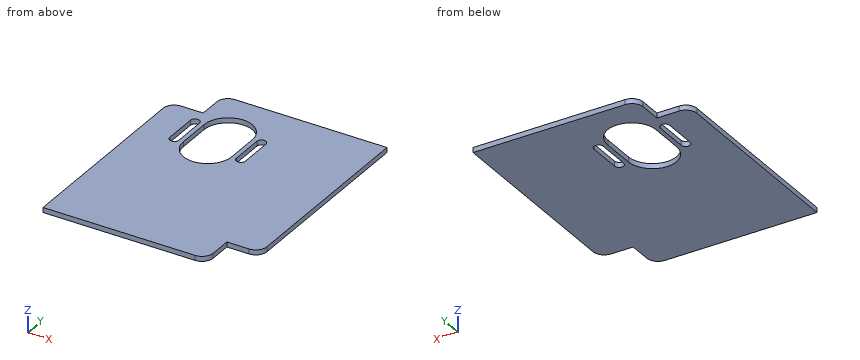
```python
from build123d import *

# Parameters (mm, degrees)
SKETCH1_W           = 118.275
SKETCH1_H           = 143.74
BOSS_EXTRUDE1_DEPTH = 3
CUT_EXTRUDE1_DEPTH  = 3
SKETCH3_W           = 20
SKETCH3_H           = 20
CUT_EXTRUDE2_DEPTH  = 10
FILLET1_R           = 6.7


with BuildPart() as part:
    # Sketch1 → Boss-Extrude1 (new body)
    with BuildSketch(Plane.XY):
        with Locations((59.1375, 71.87)):
            Rectangle(SKETCH1_W, SKETCH1_H)
    extrude(amount=BOSS_EXTRUDE1_DEPTH)

    # Sketch2 → Cut-Extrude1 (cut)
    with BuildSketch(Plane.XY.offset(3)):
        with BuildLine():
            Line((55.5, 114.05), (55.5, 94.05))
            ThreePointArc((55.5, 94.05), (41, 79.55), (26.5, 94.05))
            Line((26.5, 94.05), (26.5, 114.05))
            ThreePointArc((26.5, 114.05), (41, 128.55), (55.5, 114.05))
        make_face()
        with BuildLine():
            Line((63.75, 114.05), (63.75, 94.05))
            ThreePointArc((63.75, 94.05), (61, 91.3), (58.25, 94.05))
            Line((58.25, 94.05), (58.25, 114.05))
            ThreePointArc((58.25, 114.05), (61, 116.8), (63.75, 114.05))
        make_face()
        with BuildLine():
            Line((23.75, 114.05), (23.75, 94.05))
            ThreePointArc((23.75, 94.05), (21, 91.3), (18.25, 94.05))
            Line((18.25, 94.05), (18.25, 114.05))
            ThreePointArc((18.25, 114.05), (21, 116.8), (23.75, 114.05))
        make_face()
    extrude(amount=-CUT_EXTRUDE1_DEPTH, mode=Mode.SUBTRACT)

    # Sketch3 → Cut-Extrude2 (cut)
    with BuildSketch(Plane.XY.offset(3)):
        with Locations((10, 133.74)):
            Rectangle(SKETCH3_W, SKETCH3_H)
        with Locations((108.275, 10)):
            Rectangle(SKETCH3_W, SKETCH3_H)
    extrude(amount=-CUT_EXTRUDE2_DEPTH, mode=Mode.SUBTRACT)

    # Fillet1
    fillet1_edges = [part.edges().sort_by_distance(p)[0] for p in [
        (0, 123.74, 1.5),
        (20, 143.74, 1.5),
        (118.275, 20, 1.5),
        (98.275, 0, 1.5),
    ]]
    fillet(fillet1_edges, radius=FILLET1_R)


solid = part.part
```
For this review, take the finished solid that the model builds, in its own axes (mm). Round coordinates to 2 decimals unless told otherwise and drop trailing zeros. Write each loop counter-clockwise with the first axis right and the second up, starting at its lowest first coordinate (ties: lowest second). Pieces come first, ordered by that corner, then holes. Notation, with made-up numbers: (73, 84) - (112, 84) arc R21 ccw to (112, 92) - close; hole circle Ø3 at (81.5, -24). An arc over 180 degrees is marked (long way). Answer as a JSON object with one key per item and string values.
1. We need section A-A on x = 41. Give the boundary of the cut face in (y, z), then the cut area to 3 significant figures.
Response values:
{"outline": "(0, 0) - (79.55, 0) - (79.55, 3) - (0, 3) - close; (128.55, 0) - (143.74, 0) - (143.74, 3) - (128.55, 3) - close", "area": "284 mm2"}
2. We need section B-B on z = 2.4. Give the boundary of the cut face in (x, y) (3 decimals).
Response values:
{"outline": "(0, 0) - (91.575, 0) arc R6.7 ccw to (98.275, 6.7) - (98.275, 20) - (111.575, 20) arc R6.7 ccw to (118.275, 26.7) - (118.275, 143.74) - (26.7, 143.74) arc R6.7 ccw to (20, 137.04) - (20, 123.74) - (6.7, 123.74) arc R6.7 ccw to (0, 117.04) - close; hole (18.25, 94.05) arc R2.75 ccw to (23.75, 94.05) - (23.75, 114.05) arc R2.75 ccw to (18.25, 114.05) - close; hole (26.5, 94.05) arc R14.5 ccw to (55.5, 94.05) - (55.5, 114.05) arc R14.5 ccw to (26.5, 114.05) - close; hole (58.25, 94.05) arc R2.75 ccw to (63.75, 94.05) - (63.75, 114.05) arc R2.75 ccw to (58.25, 114.05) - close"}
3. To check wall thickness, follow line 1 along X through (y, z) = (109.5, 2.45) (3 decimals); line 2 along Y through (x, z) = (40.5, 1.8); line 3 along X through (y, z) = (88, 1.9) (3 decimals). State the ranges of each line that lie inside material, in increasing order.
Response values:
{"line 1": "x = 0 to 18.25, 23.75 to 26.5, 55.5 to 58.25, 63.75 to 118.275", "line 2": "y = 0 to 79.56, 128.54 to 143.74", "line 3": "x = 0 to 27.822, 54.178 to 118.275"}
4. We need section C-C on x = 61. Give the boundary of the cut face in (y, z), then the cut area to 3 significant figures.
Response values:
{"outline": "(0, 0) - (91.3, 0) - (91.3, 3) - (0, 3) - close; (116.8, 0) - (143.74, 0) - (143.74, 3) - (116.8, 3) - close", "area": "355 mm2"}
5. For pin 1 Ø8 at (x, y) = (103.5, 119.5) entering from -Z, flat-tipped, find the tip position at first contact; note if it passes through.
Response values:
{"pin 1": "stops at z = 0"}
